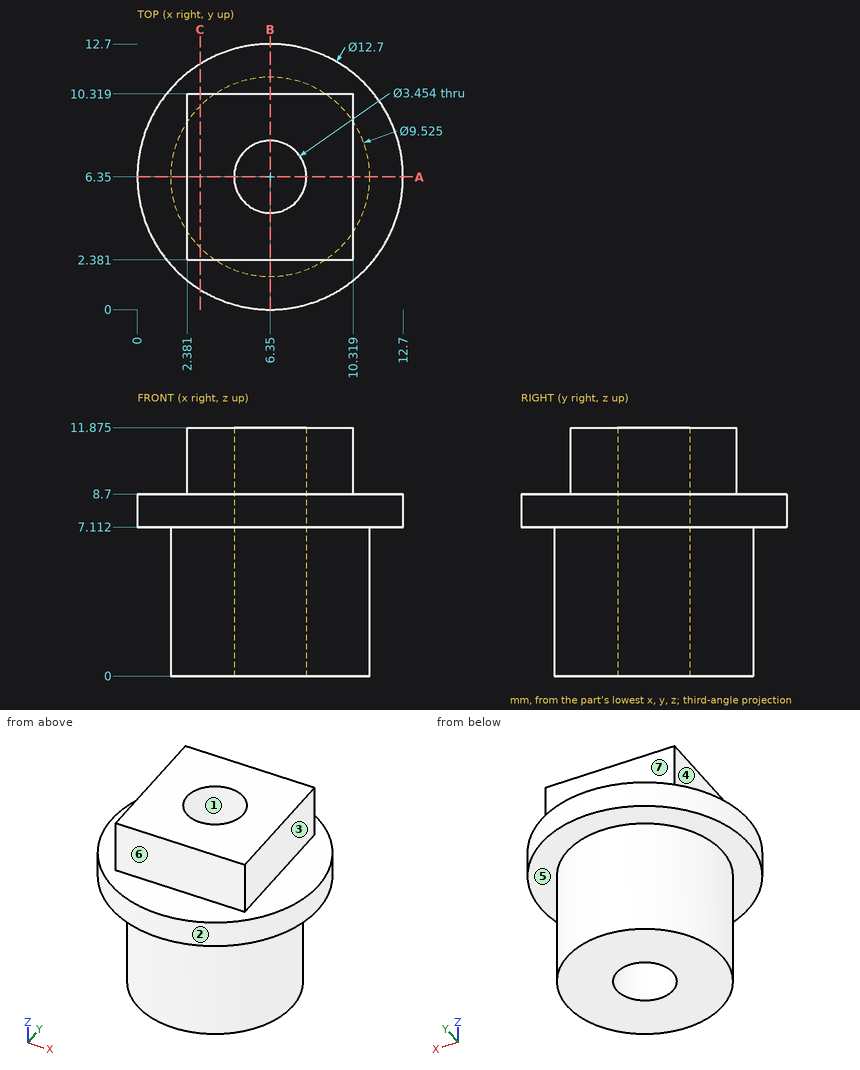
Answer from the drawing. Dimensions are ordinates in mm from the lowest x, y and z of the part. A direction names the side the tool comes from. Give positions to 0.01 mm unless a question says otherwise; leave off trailing zeros. Write each loop counter-clockwise with the first axis right and the second up, starting at its lowest first coordinate (ties: lowest second). Pieces come first, ordered by that corner, then holes. Notation, with made-up numbers: (-16.75, -5.75) - (-11.75, -5.75) arc R13 cw to (-11.75, 4.25) - close; hole circle Ø1 at (62.5, -6). An arc over 180 degrees is marked (long way). Answer in a Markdown table with one row per item. Add a question column.
Item 1: A tool of negligible diameter and unlimited length cuts with its end or side. For the marked faces 5, 6 and 7, from which of +Z, -Z, +X, -X, +Y, -Y can it reach the whole face along a straight path? Write none if from no direction.
Item 2: Flat-ended cylindrical pins translate along their axes: P1, Ø1, axis at x = 5, z = 9.5, coming from the -Y side; P2, Ø2, axis at x = 8.5, z = 9.5, coming from the -Y side; P3, Ø1, axis at y = 7.5, z = 3.5, coming from the +X side; P4, Ø5.5, axis at x = 6.35, y = 6.35, coming from the +Z side (1 decimal). Find the tip coordinate at first contact, or state that the pin passes through.
Item 3: Section C-C, the plane x = 3 is taken. Write down the section's boundary in (y, z) (1 decimal).
Item 4: Find the intervals of material crossed by L1, parallel to Y at x = 6.35, z = 4.5; L2, parallel to Y at x = 6.35, z = 8.5; L3, parallel to Y at x = 3.75, z = 10.5, in increasing order.
Item 5: Section A-A, the plane y = 6.35 is taken. Write down the section's boundary in (x, z) (1 decimal).
Item 6: Determine the mould class of the marked faces 1, 2, 3 and 4 for opening direction X: pulls with the +X half, pulls with the -X half, needs draft (parallel to the pull), parting line crosses it, or undercut.
Recorded:
| question | item | result |
|---|---|---|
| 1 | face 5 | -Z |
| 1 | face 6 | +Z, +X, -X, -Y |
| 1 | face 7 | +Z, +X, -X, +Y |
| 2 | P1 | stops at y = 2.38 |
| 2 | P2 | stops at y = 0.19 |
| 2 | P3 | stops at x = 11.07 |
| 2 | P4 | stops at z = 11.9 |
| 3 | outline | (1, 7.1) - (3, 7.1) - (3, 0) - (9.7, 0) - (9.7, 7.1) - (11.7, 7.1) - (11.7, 8.7) - (10.3, 8.7) - (10.3, 11.9) - (2.4, 11.9) - (2.4, 8.7) - (1, 8.7) - close |
| 4 | L1 | y = 1.59 to 4.62, 8.08 to 11.11 |
| 4 | L2 | y = 0 to 4.62, 8.08 to 12.7 |
| 4 | L3 | y = 2.38 to 10.32 |
| 5 | outline | (0, 7.1) - (1.6, 7.1) - (1.6, 0) - (4.6, 0) - (4.6, 11.9) - (2.4, 11.9) - (2.4, 8.7) - (0, 8.7) - close; (8.1, 0) - (11.1, 0) - (11.1, 7.1) - (12.7, 7.1) - (12.7, 8.7) - (10.3, 8.7) - (10.3, 11.9) - (8.1, 11.9) - close |
| 6 | face 1 | undercut |
| 6 | face 2 | parting line crosses it |
| 6 | face 3 | pulls with the +X half |
| 6 | face 4 | pulls with the -X half |
